```python
from build123d import *

# Parameters (mm, degrees)
F1_DEPTH = 50
F2_T     = -2.5


with BuildPart() as f1:
    # F0 (on Top) → F1 (new body)
    with BuildSketch(Plane.XY):
        with BuildLine():
            ThreePointArc((49.060916242, 80.7666611337), (-78.1512140744, 59.8120363605), (-101.6678459079, -66.9514853097))
            Line((-101.6678459079, -66.9514853097), (-101.6678459079, -103.9241496063))
            Line((-101.6678459079, -103.9241496063), (146.1859323948, -103.9241496063))
            Line((146.1859323948, -103.9241496063), (146.1859323948, -66.9514853097))
            ThreePointArc((146.1859323948, -66.9514853097), (210.5659380979, 32.5726496486), (112.5656791895, 99.2493909263))
            Line((112.5656791895, 99.2493909263), (49.060916242, 80.7666611337))
        make_face()
        Polygon((-20.3918665088, -18.0957990914), (-36.9947273911, 0.6663483047), (-46.9947273911, 0.6663483047), (-46.9947273911, 14.8120262139), (-36.9947273911, 14.8120262139), (-36.9947273911, 40.4454148785), (-10.7651253298, 40.4454148785), (-10.7090268836, 16.9306674714), (-0.5355780579, 16.9549379711), (-0.5039027498, 3.6776206944), (-10.5038742928, 3.6537640543), (-10.3919994277, -18.0442397964), align=None, mode=Mode.SUBTRACT)
    extrude(amount=F1_DEPTH)

    # F2
    f2_openings = [f1.faces().sort_by_distance(p)[0] for p in [
        (49.091744, -6.264169, 50),
    ]]
    offset(amount=F2_T, openings=f2_openings, kind=Kind.INTERSECTION)


solid = f1.part
```
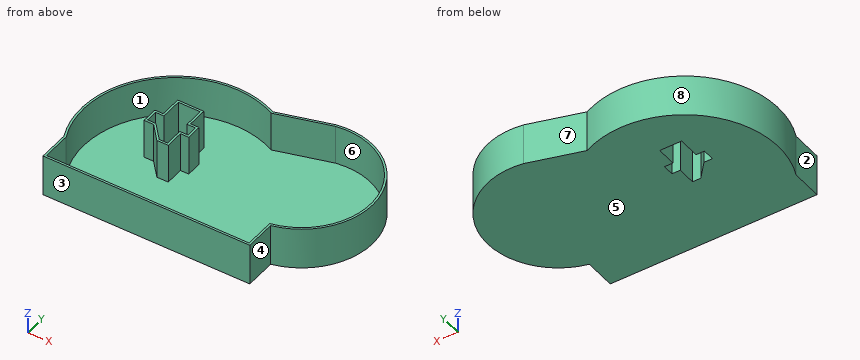
Geometry check sheet. Reference: the model listing, model coordinates, mm. Face numbers are marked on the shaded views. A direction names the side the tool comes from. Round coordinates to 2 decimals unless told otherwise and drop trailing zeros. Order: outer loops, then holes, each group sorted by start corner. A loop starts at its lowest first (then second) coordinate and runs counter-clockwise, first axis right, second up. Notation, with made-up numbers: (1, 48) -> (31, 48) arc R22 ccw to (31, 79) -> close; hole circle Ø6 at (76.5, -8). An arc over 180 degrees is marked (long way). Return JSON: item names as keys, results as strings. Group by question number.
Q1. Section check D-D, the plane x = 67. Record the boundary of the cut face in (y, z), plus the area to 3 significant figures.
Q2. Section check B-B, the plane y = 36. Record the boundary of the cut face in (x, z).
Q3. Release check for a two-part mould opening along X. For the marked faces 1, 2 and 3 record: released by +X, released by -X, zero draft, split by the parting line, or undercut.
Q4. Gauge pin test, flat ends, axial feed: pin 1 (14 mm diameter, centred on x = 70, z = 17.5, fed in from +Y); pin 2 (18 mm diameter, centred on y = -77.5, z = 19.5, fed in from -X); pin 3 (10 mm diameter, centred on x = 159, z = 37.5, fed in from +Y). Record the tip position at first contact, or that the pin passes through.
Q5. Section check A-A, the plane z = 12. Count the separate pieces of the cut face and the enclosed holes in it, plus the area to 3 significant figures.
Q6. Material ranges on probe 1 along X at (y, z) = (3.5, 22); probe 2 along Y at (x, z) = (-28, 48); probe 3 along Y at (x, z) = (-49, 31.5), recorded low to high. Write a range as from..to.
Q7. Section check C-C, the plane y = -71. Record the boundary of the cut face in (x, z), plus the area to 3 significant figures.
Q8. Tool access check on the marked faces 4, 5, 6, 7 and 8. Record the directions out of +Z, -Z, +X, -X, +Y, -Y that give a thin tool (end or side, any length) a straight path to the whole face; none if there is none.
Numbers:
{
 "1": {"outline": "(-103.92, 0) -> (85.99, 0) -> (85.99, 50) -> (83.38, 50) -> (83.38, 2.5) -> (-101.42, 2.5) -> (-101.42, 50) -> (-103.92, 50) -> close", "area": "717 mm^2"},
 "2": {"outline": "(-96.66, 0) -> (-36.99, 0) -> (-36.99, 50) -> (-39.49, 50) -> (-39.49, 2.5) -> (-93.76, 2.5) -> (-93.76, 50) -> (-96.66, 50) -> close; (-10.75, 0) -> (209.8, 0) -> (209.8, 50) -> (207.22, 50) -> (207.22, 2.5) -> (-8.25, 2.5) -> (-8.25, 50) -> (-10.75, 50) -> close"},
 "3": {"face 1": "undercut", "face 2": "released by -X", "face 3": "zero draft"},
 "4": {"pin 1": "y = 88.9", "pin 2": "x = -101.67", "pin 3": "y = 96.3"},
 "5": {"separate pieces": "2", "enclosed holes": "2", "area": "2,820 mm^2"},
 "6": {"probe 1": "-109.26..-106.7, -49.49..-46.99, -10.5..2, 208.83..211.36", "probe 2": "-103.92..-101.42, -13.27..-9.5, 40.45..42.95, 85.64..88.23", "probe 3": "-103.92..-101.42, -1.83..17.31, 77.64..80.43"},
 "7": {"outline": "(-101.67, 0) -> (146.19, 0) -> (146.19, 50) -> (143.69, 50) -> (143.69, 2.5) -> (-99.17, 2.5) -> (-99.17, 50) -> (-101.67, 50) -> close", "area": "857 mm^2"},
 "8": {"face 4": "+Z, -Z, +X, -Y", "face 5": "-Z, +X, -X, +Y, -Y", "face 6": "+Z", "face 7": "+Z, -Z, +Y", "face 8": "+Z, -Z"}
}
